Check sheet for the modelled part. Datum: model origin and axes. Units: mm. A direction names the side the tool comes from. Round coordinates to 2 decimals unless told otherwise and drop trailing zeros. Order: outer loops, then holes, each group sorted by start corner. A loop starts at its lowest first (then second) coordinate and runs counter-clockwise, first axis right, second up.
(1) Sectioned sample at C-C, the plane y = -19.5. Enter the section's corners in (x, z).
(2) Sectioned sample at A-A, the plane z = 13.25. Enter the section's corners in (x, y), and give its area (3 significant figures).
(3) Sectioned sample at D-D, the plane x = -19. Enter the section's corners in (y, z).
(4) Mould release check, pull along X, two halves, no side actions. Record for faces 1 (the flat face through (-11, -25, 23)), 2 (the flat face through (14.5, -12, 8)), 3 (the flat face through (13.5, -12, 8)), 4 (the flat face through (-14.5, -12, 8)): released by +X, released by -X, zero draft, split by the parting line, or undercut.
(5) Thickness scan on probe 1 along X at (y, z) = (-17, 9.5); probe 2 along Y at (x, z) = (-21, 0.55); probe 3 along Z at (x, y) = (-21.5, -16.5). Record the ranges inside material, lowest first.
(6) Depth check by flat-ended pin: pin 1 (5 mm diameter, centred on y = -10.5, z = 22, fed in from -X); pin 2 (4 mm diameter, centred on x = 20, y = -10, fed in from +Z); pin 3 (6 mm diameter, centred on y = -8.5, z = 7, fed in from +X). Enter the tip coordinate at first touch or a pass-through.
(7) Tool access check on faces 5 (the flat face through (-23, -12, 1)), 6 (the flat face through (24, -12, 1)), 7 (the flat face through (-13.5, -12, 7)). Record the directions out of +Z, -Z, +X, -X, +Y, -Y that give a thin tool (end or side, any length) a straight path to the whole face; none if there is none.
(8) Sectioned sample at B-B, the plane x = 21. Enter the section's corners in (y, z), and give its area (3 significant figures).
```python
from build123d import *

# Parameters (mm, degrees)
F1_DEPTH = 25
F2_R     = 1
F3_DEPTH = 25
F4_R     = 1
F5_R     = 1


with BuildPart() as f1:
    # F0 (on Front) → F1 (new body)
    with BuildSketch(Plane.XZ):
        with BuildLine():
            ThreePointArc((-13.5, 13.85), (-9.545942, 23.395942), (0, 27.35))
            Line((0, 27.35), (0, 28.35))
            ThreePointArc((0, 28.35), (-10.253048, 24.103048), (-14.5, 13.85))
            Line((-14.5, 13.85), (-14.5, 1))
            Line((-14.5, 1), (-28.5, 1))
            Line((-28.5, 1), (-28.5, 0))
            Line((-28.5, 0), (-13.5, 0))
            Line((-13.5, 0), (-13.5, 13.85))
        make_face()
        with BuildLine():
            Line((0, 28.35), (0, 27.35))
            ThreePointArc((0, 27.35), (9.545942, 23.395942), (13.5, 13.85))
            Line((13.5, 13.85), (13.5, 0))
            Line((13.5, 0), (28.5, 0))
            Line((28.5, 0), (28.5, 1))
            Line((28.5, 1), (14.5, 1))
            Line((14.5, 1), (14.5, 13.85))
            ThreePointArc((14.5, 13.85), (10.253048, 24.103048), (0, 28.35))
        make_face()
    extrude(amount=F1_DEPTH)

    # F2 (on face) → F3 (cut)
    with BuildSketch(Plane.XY.offset(1)):
        with Locations((-21, -12.5)):
            Circle(F2_R)
        with Locations((21, -12.5)):
            Circle(F2_R)
    extrude(amount=-F3_DEPTH, mode=Mode.SUBTRACT)

    # F4
    f4_edges = [f1.edges().sort_by_distance(p)[0] for p in [
        (14.5, -12.5, 1),
        (13.5, -12.5, 0),
    ]]
    fillet(f4_edges, radius=F4_R)

    # F5
    f5_edges = [f1.edges().sort_by_distance(p)[0] for p in [
        (-14.5, -12.5, 1),
        (-13.5, -12.5, 0),
    ]]
    fillet(f5_edges, radius=F5_R)


solid = f1.part
```
Derived:
1. outline: (-28.5, 0) - (-14.5, 0) arc R1 ccw to (-13.5, 1) - (-13.5, 13.85) arc R13.5 cw to (0, 27.35) arc R13.5 cw to (13.5, 13.85) - (13.5, 1) arc R1 ccw to (14.5, 0) - (28.5, 0) - (28.5, 1) - (15.5, 1) arc R1 cw to (14.5, 2) - (14.5, 13.85) arc R14.5 ccw to (0, 28.35) arc R14.5 ccw to (-14.5, 13.85) - (-14.5, 2) arc R1 cw to (-15.5, 1) - (-28.5, 1) - close
2. outline: (-14.5, -25) - (-13.5, -25) - (-13.5, 0) - (-14.5, 0) - close; (13.5, -25) - (14.5, -25) - (14.5, 0) - (13.5, 0) - close
2. area: 50.0 mm2
3. outline: (-25, 0) - (0, 0) - (0, 1) - (-25, 1) - close
4. face 1: zero draft
4. face 2: released by +X
4. face 3: undercut
4. face 4: released by -X
5. probe 1: x = -14.5 to -13.5, 13.5 to 14.5
5. probe 2: y = -25 to -13.5, -11.5 to 0
5. probe 3: z = 0 to 1
6. pin 1: stops at x = -13.35
6. pin 2: stops at z = 1
6. pin 3: stops at x = 14.5
7. face 5: +Z, -X, +Y, -Y
7. face 6: +Z, +X, +Y, -Y
7. face 7: -Z, +Y, -Y
8. outline: (-25, 0) - (-13.5, 0) - (-13.5, 1) - (-25, 1) - close; (-11.5, 0) - (0, 0) - (0, 1) - (-11.5, 1) - close
8. area: 23.0 mm2
